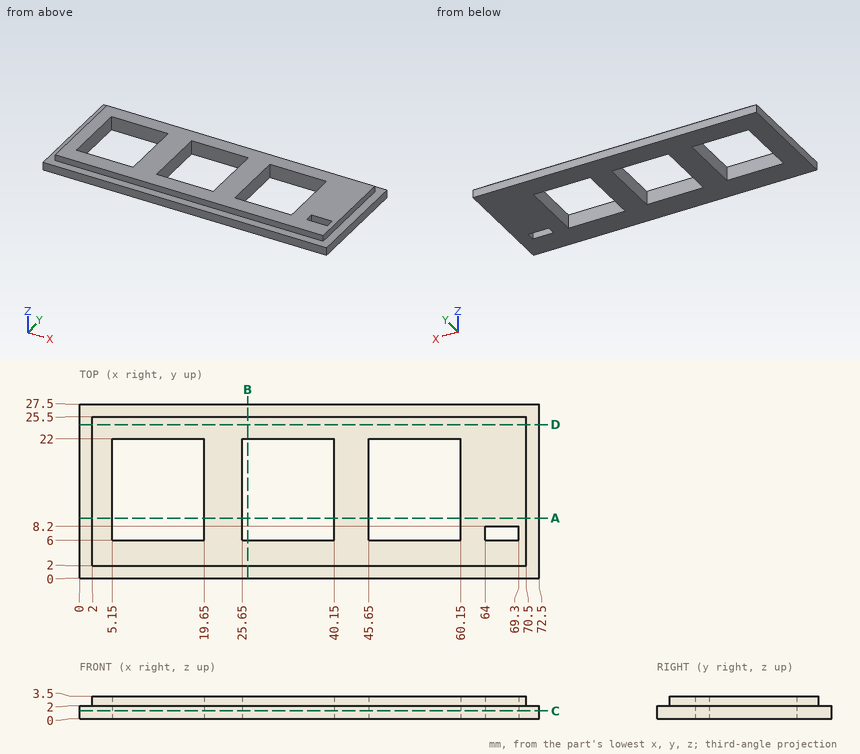
Source: three-view drawing plus pictorial views. Frame: mm from the lowest corner of the part. Round coordinates to 2 decimals unless told otherwise and drop trailing zeros. Write each loop counter-clockwise with the first axis right and the second up, starting at its lowest first coordinate (ties: lowest second). Pieces come first, ordered by that corner, then holes. Notation, with made-up numbers: M -5.5,70.25 L 15.5,70.25 A27 ccw 15.5,91.25 Z; hole C 72,17.25 d3. An arc over 180 degrees is marked long. One line per item, written item: value. Start each with the question number.
Item 1: Section query C-C (z = 1.2). Return the cut outline in (x, y).
Item 2: Ray query, L1, parallel to X at y = 21.75, z = 0.6; L2, parallel to X at y = 21.75, z = 2.45; L3, parallel to Y at x = 16.5, z = 2.1. Return the intervals inside material, ascending. Write a range as from..to.
Item 3: Section query A-A (y = 9.5). Return the cut outline in (x, z), plus the area to 3 significant figures.
Item 4: Section query B-B (x = 26.5). Return the cut outline in (y, z), plus the area to 4 significant figures.
Item 5: Pin query (flat end, axial travel): pin 1 (1.6 mm diameter, centred on x = 48.5, z = 3, fed in from +Y). Return the tip coordinate at first contact, or that it passes through.
Item 6: Section query D-D (y = 24.25). Return the cut outline in (x, z).
Result set:
1. outline: M 0,0 L 72.5,0 L 72.5,27.5 L 0,27.5 Z; hole M 5.15,6 L 19.65,6 L 19.65,22 L 5.15,22 Z; hole M 25.65,6 L 40.15,6 L 40.15,22 L 25.65,22 Z; hole M 45.65,6 L 60.15,6 L 60.15,22 L 45.65,22 Z; hole M 64,6 L 69.3,6 L 69.3,8.2 L 64,8.2 Z
2. L1: x = 0..5.15, 19.65..25.65, 40.15..45.65, 60.15..72.5
2. L2: x = 2..5.15, 19.65..25.65, 40.15..45.65, 60.15..70.5
2. L3: y = 2..6, 22..25.5
3. outline: M 0,0 L 5.15,0 L 5.15,3.5 L 2,3.5 L 2,2 L 0,2 Z; M 19.65,0 L 25.65,0 L 25.65,3.5 L 19.65,3.5 Z; M 40.15,0 L 45.65,0 L 45.65,3.5 L 40.15,3.5 Z; M 60.15,0 L 72.5,0 L 72.5,2 L 70.5,2 L 70.5,3.5 L 60.15,3.5 Z
3. area: 95.5 mm²
4. outline: M 0,0 L 6,0 L 6,3.5 L 2,3.5 L 2,2 L 0,2 Z; M 22,0 L 27.5,0 L 27.5,2 L 25.5,2 L 25.5,3.5 L 22,3.5 Z
4. area: 34.25 mm²
5. pin 1: stops at y = 25.5
6. outline: M 0,0 L 72.5,0 L 72.5,2 L 70.5,2 L 70.5,3.5 L 2,3.5 L 2,2 L 0,2 Z
